Geometry check sheet. Reference: the model listing, model coordinates, mm. Face numbers are marked on the shaded views. Coordinates: 2 decimals unless noted, no trailing zeros. Write each loop counter-clockwise with the first axis right and the second up, starting at its lowest first coordinate (ties: lowest second). Pieces come first, ordered by that corner, then holes.
from build123d import *

# Parameters (mm, degrees)
SKETCH1_W          = 8
SKETCH1_H          = 2
CHAMFER1_SIZE      = 0.525
CUT_EXTRUDE2_DEPTH = 1.54


with BuildPart() as part:
    # Sketch1 → Revolve1 (revolve)
    with BuildSketch(Plane(origin=(0, 0, 0), x_dir=(0, 0, -1), z_dir=(1, 0, 0))):
        with Locations((6.2, 1)):
            Rectangle(SKETCH1_W, SKETCH1_H)
    revolve(axis=Axis((0, 0, -10.2), (0, 0, 1)))

    # Chamfer1
    chamfer1_edges = [part.edges().sort_by_distance(p)[0] for p in [
        (0, -2, -10.2),
    ]]
    chamfer(chamfer1_edges, length=CHAMFER1_SIZE)

    # Sketch7 → Revolve2 (revolve)
    with BuildSketch(Plane(origin=(0, 0, 0), x_dir=(0, 0, -1), z_dir=(1, 0, 0)), mode=Mode.PRIVATE) as revolve2_sk:
        with BuildLine():
            Line((1.87, 3.8), (2.2, 3.8))
            Line((2.2, 3.8), (2.2, 0))
            Line((2.2, 0), (0, 0))
            Line((0, 0), (0, 2))
            ThreePointArc((0, 2), (0.793500147, 3.047002626), (1.87, 3.8))
        make_face()
    revolve(revolve2_sk.sketch.rotate(Axis((0, 0, 0), (0, 0, -1)), 180), axis=Axis((0, 0, 0), (0, 0, -1)))

    # Sketch5 → Cut-Extrude2 (cut)
    with BuildSketch(Plane.XY):
        Polygon((1.25, -0.721687836), (1.25, 0.721687836), (0, 1.443375673), (-1.25, 0.721687836), (-1.25, -0.721687836), (0, -1.443375673), align=None)
    extrude(amount=-CUT_EXTRUDE2_DEPTH, mode=Mode.SUBTRACT)

    # Cut-Extrude3 cone 1 section (on through the dimple's axis) → Cut-Extrude3 (revolve, cut)
    with BuildSketch(Plane(origin=(0, 0, 0), x_dir=(0, -1, 0), z_dir=(1, 0, 0))):
        Polygon((0, 0), (1.443375673, 0), (0, 1.443375673), align=None)
    revolve(axis=Axis((0, 0, 0), (0, 0, -1)), mode=Mode.SUBTRACT)


solid = part.part
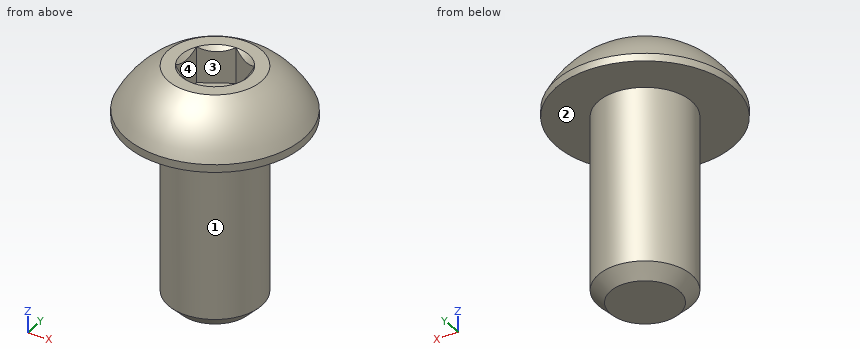
1. Sectioned sample at B-B, the plane z = -0.5. Record the boundary of the cut face in (x, y), and give its area (3 significant figures).
Computed values:
outline: circle Ø5.47 at (0, 0); hole (-1.25, -0.72) - (0, -1.44) - (1.25, -0.72) - (1.25, 0.72) - (0, 1.44) - (-1.25, 0.72) - close
area: 18.1 mm2
2. Sectioned sample at A-A, the plane y = 0. Record the boundary of the cut face in (x, z) (3 decimals), and give its area (3 significant figures).
Computed values:
outline: (-3.8, -2.2) - (-2, -2.2) - (-2, -9.675) - (-1.475, -10.2) - (1.475, -10.2) - (2, -9.675) - (2, -2.2) - (3.8, -2.2) - (3.8, -1.87) arc R4.229 ccw to (2, 0) - (1.443, 0) - (1.25, -0.193) - (1.25, -1.54) - (-1.25, -1.54) - (-1.25, -0.193) - (-1.443, 0) - (-2, 0) arc R4.229 ccw to (-3.8, -1.87) - close
area: 41.9 mm2
3. Thickness scan on line 1 along X through (y, z) = (1.25, -4.75); line 2 along X through (y, z) = (0.5, -2.5); line 3 along Z through (x, y) = (2.25, 1.75). Record the ranges inside material, lowest first.
Computed values:
line 1: x = -1.56 to 1.56
line 2: x = -1.94 to 1.94
line 3: z = -2.2 to -0.6
4. Sectioned sample at C-C, the plane z = -6.25. Record the boundary of the cut face in (x, y).
Computed values:
outline: circle Ø4 at (0, 0)
5. Gauge pin test, flat ends, axial feed: pin 1 Ø3 at (y, z) = (2, -6.5) entering from +X; pin 2 Ø1.5 at (x, y) = (-3, -3) entering from -Z; pin 3 Ø4 at (x, y) = (-2.5, -2) entering from +Z; pin 4 Ø4 at (y, z) = (3, -2.5) entering from -X. Record the tip position at first contact, or that the pin passes through.
Computed values:
pin 1: stops at x = 1.94
pin 2: stops at z = -2.2
pin 3: stops at z = 0
pin 4: stops at x = -3.66
6. Draft check along X on the marked faces 1, 2, 3 and 4. Enter one of: released by +X, released by -X, zero draft, split by the parting line, or undercut.
Computed values:
face 1: split by the parting line
face 2: zero draft
face 3: undercut
face 4: undercut
7. Sectioned sample at D-D, the plane x = 3. Record the boundary of the cut face in (y, z), and give its area (3 significant figures).
Computed values:
outline: (-2.33, -2.2) - (2.33, -2.2) - (2.33, -1.87) arc R2.98 ccw to (-2.33, -1.87) - close
area: 5.19 mm2
